from build123d import *

# Parameters (mm, degrees)
BASECHANNELSE_DEPTH = 127


with BuildPart() as part:
    # Sketch1 → BaseChannelse (new, symmetric)
    with BuildSketch(Plane.XY):
        with BuildLine():
            Line((0, 0), (0, 26.924))
            Line((0, 26.924), (31.75, 26.924))
            Line((31.75, 26.924), (31.75, 23.749))
            Line((31.75, 23.749), (4.76504, 23.749))
            ThreePointArc((4.76504, 23.749), (4.763243949, 23.748256051), (4.7625, 23.74646))
            Line((4.7625, 23.74646), (4.7625, 3.17754))
            ThreePointArc((4.7625, 3.17754), (4.763243949, 3.175743949), (4.76504, 3.175))
            Line((4.76504, 3.175), (31.75, 3.175))
            Line((31.75, 3.175), (31.75, 0))
            Line((31.75, 0), (0, 0))
        make_face()
    extrude(amount=BASECHANNELSE_DEPTH, both=True)


solid = part.part
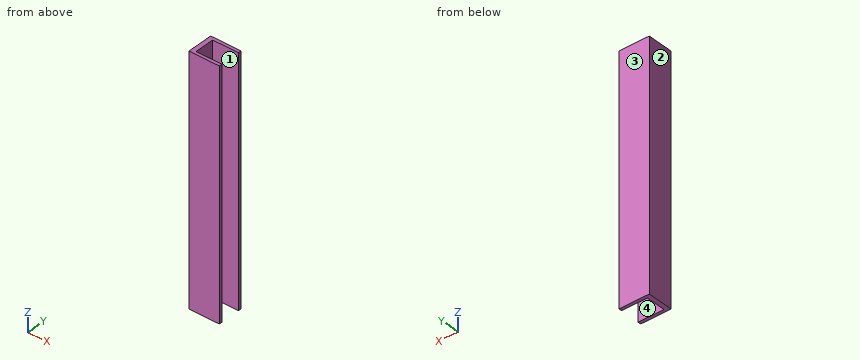
Here's how the part is built. I have some questions about the finished solid (model axes, mm). Face numbers are marked on the shaded views. Give positions to 0.01 mm unless a question says otherwise; leave off trailing zeros. Loops run counter-clockwise (first coordinate to the right, second up) from the corner with the lowest first, then second, coordinate; pieces in that order, holes last. Notation, with made-up numbers: (21, 66) -> (32, 66) arc R33 ccw to (32, 96) -> close; hole circle Ø6 at (-9.5, -29). An arc over 180 degrees is marked (long way). One line per item, written item: value.
Q1. I'm going to push flat-ended pins straight in: pin 1 Ø5 at (x, y) = (20.5, 21) entering from -Z; pin 2 Ø5 at (y, z) = (11.5, -27.5) entering from +X; pin 3 Ø13.5 at (x, z) = (20, -8) entering from -Y. Where does each tip first touch, or does it pass through?
Answers follow:
pin 1: through
pin 2: x = 4.76
pin 3: y = 0
Q2. Suppose I cut it at A-A on x = 15. Please give me the cut outline in (y, z) (3 decimals), then the cut area to 3 significant figures.
Answers follow:
outline: (0, -127) -> (3.175, -127) -> (3.175, 127) -> (0, 127) -> close; (23.749, -127) -> (26.924, -127) -> (26.924, 127) -> (23.749, 127) -> close
area: 1,610 mm^2
Q3. If I drill on line 1 along Y through (x, z) = (25, 78.5) (3 decimals); line 2 along X through (y, z) = (17.25, 7.5), over which ranges is the centre line in solid material (lowest first)?
Answers follow:
line 1: 0 to 3.175, 23.749 to 26.924
line 2: 0 to 4.76
Q4. Suppose I cut it at C-C on y = 6.5. Please give me the cut outline in (x, z), then the cut area to 3 significant figures.
Answers follow:
outline: (0, -127) -> (4.76, -127) -> (4.76, 127) -> (0, 127) -> close
area: 1,210 mm^2
Q5. We'd pull the mould along Y, two halves only. Please class the marked faces 1, 2, 3 and 4: pulls with the +Y half, pulls with the -Y half, needs draft (parallel to the pull), parting line crosses it, or undercut.
Answers follow:
face 1: undercut
face 2: needs draft
face 3: pulls with the +Y half
face 4: undercut
